Verification items for this drawing (mm, ordinates from the low corner). Give positions to 0.01 mm unless a question says otherwise; leave off trailing zeros. Loops run counter-clockwise (first coordinate to the right, second up) from the corner with the lowest first, then second, coordinate; pieces in that order, holes last. Notation, with made-up numbers: (65.25, -23.75) -> (119.25, -23.75) arc R24 cw to (119.25, -6.75) -> close; hole circle Ø10 at (9.25, 54.5). An arc over 180 degrees is marked (long way). Answer as CSV lines item,"result". Start each with the question number.
(1) Section check B-B on x = 34. Enter the section's corners in (y, z).
(2) Gauge pin test, flat ends, axial feed: pin 1 Ø4 at (y, z) = (5.5, 42.5) entering from -X; pin 2 Ø8 at (x, z) = (19.5, 42) entering from +Y; pin 3 Ø0.5 at (x, y) = (20, 11) entering from +Z. Record the tip position at first contact, or that the pin passes through.
(3) Material ranges on line 1 (Y direction, x = 46.5, z = 9); line 2 (Y direction, x = 48.5, z = 54.5); line 3 (Z direction, x = 22, y = 10.75), recorded low to high. Write a range as from..to.
(4) Section check D-D on y = 7. Enter the section's corners in (x, z).
(5) Section check A-A on z = 11.5. Enter the section's corners in (x, y), plus the area to 3 significant figures.
(6) Release check for a two-part mould opening along Y. For the marked faces 1, 2 and 3 record: pulls with the +Y half, pulls with the -Y half, needs draft (parallel to the pull), parting line crosses it, or undercut.
(7) Section check C-C on z = 35. Enter the section's corners in (x, y), plus the area to 3 significant figures.
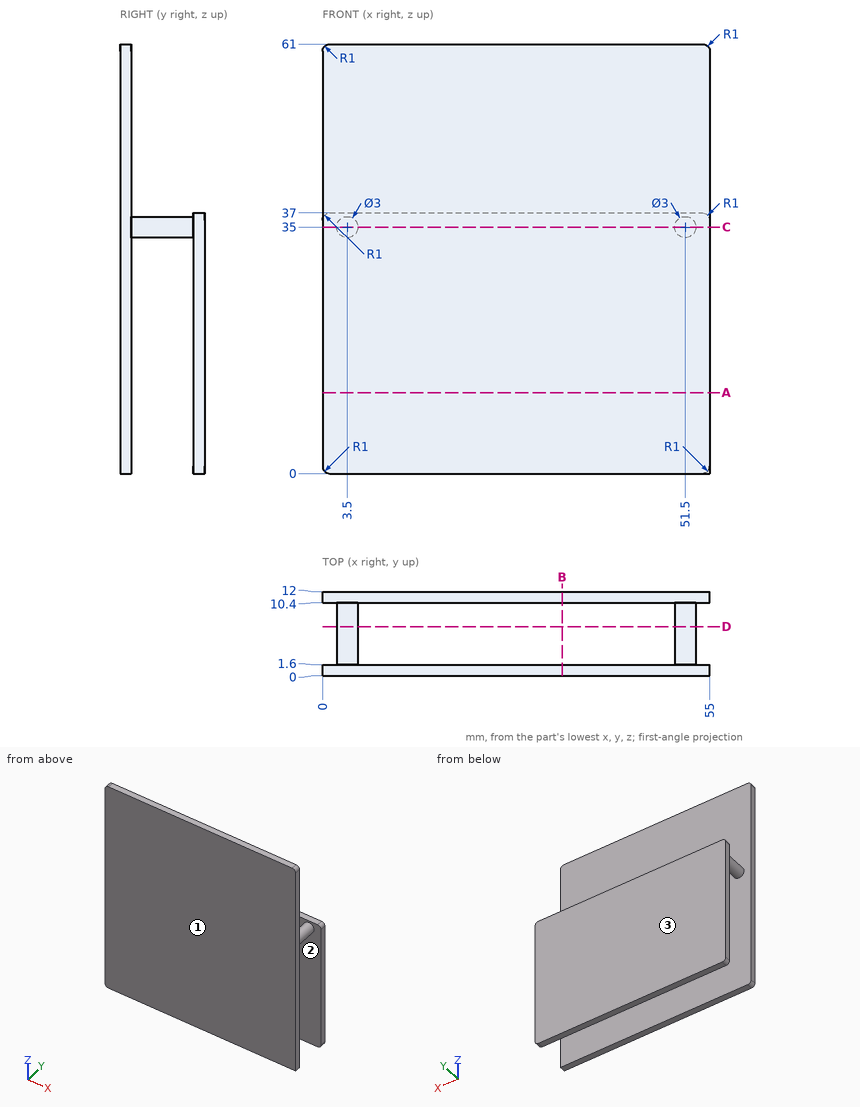
Working result:
1,outline,"(0, 0) -> (1.6, 0) -> (1.6, 61) -> (0, 61) -> close; (10.4, 0) -> (12, 0) -> (12, 37) -> (10.4, 37) -> close"
2,pin 1,"passes through"
2,pin 2,"stops at y = 1.6"
2,pin 3,"stops at z = 37"
3,line 1,"y = 0..1.6, 10.4..12"
3,line 2,"y = 0..1.6"
3,line 3,"z = 0..37"
4,outline,"circle Ø3 at (3.5, 35); circle Ø3 at (51.5, 35)"
5,outline,"(0, 0) -> (55, 0) -> (55, 1.6) -> (0, 1.6) -> close; (0, 10.4) -> (55, 10.4) -> (55, 12) -> (0, 12) -> close"
5,area,"176 mm^2"
6,face 1,"pulls with the -Y half"
6,face 2,"undercut"
6,face 3,"pulls with the +Y half"
7,outline,"(0, 0) -> (55, 0) -> (55, 1.6) -> (53, 1.6) -> (53, 10.4) -> (55, 10.4) -> (55, 12) -> (0, 12) -> (0, 10.4) -> (2, 10.4) -> (2, 1.6) -> (0, 1.6) -> close; hole (5, 1.6) -> (50, 1.6) -> (50, 10.4) -> (5, 10.4) -> close"
7,area,"229 mm^2"
